Model file for the job. Use its own axes, mm. A direction names the side the tool comes from. Give positions to 0.01 mm unless a question says otherwise; leave off trailing zeros. Loops run counter-clockwise (first coordinate to the right, second up) from the corner with the lowest first, then second, coordinate; pieces in that order, holes last. Notation, with made-up numbers: (63.25, -36) - (76.25, -36) arc R20 cw to (76.25, -2) - close; hole circle Ø10 at (69.25, 4). An arc over 180 degrees is marked (long way). Answer as CSV lines item,"result". Start each with the question number.
Item 1: Tool access for faces 1 (the flat face through (12.5, 0, 19)), 2 (the flat face through (14.5, 0, 18)): list every direction of +Z, -Z, +X, -X, +Y, -Y with a clear straight run to the whole face (end or side of a thin tool).
Item 2: Drill centre lines: L1, parallel to Y at x = 8.5, z = 3; L2, parallel to Z at x = 10.5, y = 3.5; L3, parallel to X at y = 1.5, z = 26. Where is each one in solid material? Low to high. Write a range as from..to.
Item 3: Saw through at C-C on y = 0.75. Give the cut face in (x, z), plus the area to 3 significant figures.
Item 4: Saw through at A-A on x = 1. Give the cut face in (y, z), plus the area to 3 significant figures.
Item 5: Saw through at B-B on z = 30.5. Give the cut face in (x, y), plus the area to 3 significant figures.
from build123d import *

# Parameters (mm, degrees)
F0_W     = 29
F0_H     = 24
F0_W_2   = 25
F0_H_2   = 20
F1_DEPTH = 38.1
F2_DEPTH = 2
F3_W     = 20
F3_H     = 38.1
F4_DEPTH = 2


with BuildPart() as f1:
    # F0 (on Top) → F1 (new body)
    with BuildSketch(Plane.XY):
        Rectangle(F0_W, F0_H)
        Rectangle(F0_W_2, F0_H_2, mode=Mode.SUBTRACT)
    extrude(amount=F1_DEPTH)

    # F0 (on Top) → F2 (join)
    with BuildSketch(Plane.XY):
        Rectangle(F0_W, F0_H)
        Rectangle(F0_W_2, F0_H_2, mode=Mode.SUBTRACT)
        Rectangle(F0_W_2, F0_H_2)
    extrude(amount=-F2_DEPTH)

    # F3 (on face) → F4 (cut)
    with BuildSketch(Plane(origin=(-14.5, 0, 0), x_dir=(0, -1, 0), z_dir=(-1, 0, 0))):
        with Locations((0, 19.05)):
            Rectangle(F3_W, F3_H)
    extrude(amount=-F4_DEPTH, mode=Mode.SUBTRACT)


solid = f1.part
Responses:
1,face 1,"+Z, -X"
1,face 2,"+Z, -Z, +X, +Y, -Y"
2,L1,"-12..-10, 10..12"
2,L2,"-2..0"
2,L3,"12.5..14.5"
3,outline,"(-14.5, -2) - (14.5, -2) - (14.5, 38.1) - (12.5, 38.1) - (12.5, 0) - (-14.5, 0) - close"
3,area,"134 mm2"
4,outline,"(-12, -2) - (12, -2) - (12, 38.1) - (10, 38.1) - (10, 0) - (-10, 0) - (-10, 38.1) - (-12, 38.1) - close"
4,area,"200 mm2"
5,outline,"(-14.5, -12) - (14.5, -12) - (14.5, 12) - (-14.5, 12) - (-14.5, 10) - (12.5, 10) - (12.5, -10) - (-14.5, -10) - close"
5,area,"156 mm2"
